Read the model definition and answer for the solid it produces. Units are mm, in the model's axes. A direction names the side the tool comes from. Give positions to 0.01 mm unless a question says otherwise; leave off trailing zeros. Order: outer loops, then holes, each group sorted by start corner. A loop starts at its lowest first (then second) coordinate and runs counter-clockwise, first axis right, second up. Notation, with made-up numbers: (83, 4.25) -> (106, 4.25) arc R27 ccw to (106, 40.25) -> close; hole circle Ø11 at (50.25, 14). An arc over 180 degrees is marked (long way). Use one line per item in the form item = value.
```python
from build123d import *

# Parameters (mm, degrees)
F0_W        = 22
F0_H        = 2
F1_DEPTH    = 25
F2_T1_DEPTH = 25
F2_T3_DEPTH = 35.98872287
F2_T5_DEPTH = 34.5227248018
F2_T7_DEPTH = 35


# Not quite as in the source:
# - a fillet or chamfer that OpenCascade refuses, or shapes differently, is made with other operations: its cross-section is extruded or revolved along the edge and cut away or added


with BuildPart() as f1:
    # F0 (on Top) → F1 (new body)
    with BuildSketch(Plane.XY):
        with BuildLine():
            ThreePointArc((-4.8733971724, -18.3643676722), (-18.9479647202, 1.4052163402), (-2.1111111111, 18.88235181))
            Line((-2.1111111111, 18.88235181), (-2.5, 22.360679775))
            ThreePointArc((-2.5, 22.360679775), (-21.7874934858, 5.6173950908), (-13, -18.3643676722))
            Line((-13, -18.3643676722), (-4.8733971724, -18.3643676722))
        make_face()
        with BuildLine():
            ThreePointArc((2.1111111111, 18.88235181), (14.1617638575, 12.6666666667), (19, 0))
            ThreePointArc((19, 0), (15.0597899434, -11.5845900602), (4.8733971724, -18.3643676722))
            Line((4.8733971724, -18.3643676722), (13, -18.3643676722))
            ThreePointArc((13, -18.3643676722), (19.9843688917, -10.3380365641), (22.5, 0))
            ThreePointArc((22.5, 0), (16.7705098312, 15), (2.5, 22.360679775))
            Line((2.5, 22.360679775), (2.1111111111, 18.88235181))
        make_face()
        with BuildLine():
            Line((13, -18.3643676722), (4.8733971724, -18.3643676722))
            ThreePointArc((4.8733971724, -18.3643676722), (0, -19), (-4.8733971724, -18.3643676722))
            Line((-4.8733971724, -18.3643676722), (-13, -18.3643676722))
            ThreePointArc((-13, -18.3643676722), (0, -22.5), (13, -18.3643676722))
        make_face()
        with BuildLine():
            Line((13, -26.3643676722), (13, -18.3643676722))
            ThreePointArc((13, -18.3643676722), (0, -22.5), (-13, -18.3643676722))
            Line((-13, -18.3643676722), (-13, -26.3643676722))
            Line((-13, -26.3643676722), (13, -26.3643676722))
        make_face()
        with Locations((0, -23.5643676722)):
            Rectangle(F0_W, F0_H, mode=Mode.SUBTRACT)
    extrude(amount=F1_DEPTH)

    # F2: fillet of radius 2 on 8 edges, made by hand

    # F2_s2 → F2_t1 (join)
    with BuildSketch(Plane.XY):
        with BuildLine():
            ThreePointArc((-13.7755102041, -17.79003425), (-13.2043135586, -18.490740056), (-13, -19.3713706278))
            Line((-13, -19.3713706278), (-13, -18.3643676722))
            ThreePointArc((-13, -18.3643676722), (-13.390834604, -18.0813591471), (-13.7755102041, -17.79003425))
        make_face()
        with BuildLine():
            ThreePointArc((13, -19.3713706278), (13.2043135586, -18.490740056), (13.7755102041, -17.79003425))
            ThreePointArc((13.7755102041, -17.79003425), (13.390834604, -18.0813591471), (13, -18.3643676722))
            Line((13, -18.3643676722), (13, -19.3713706278))
        make_face()
    extrude(amount=F2_T1_DEPTH)

    # F2_s4 → F2_t3 (cut)
    with BuildSketch(Plane.XY.offset(-5.494361435)):
        with BuildLine():
            ThreePointArc((-2.2669117515, 20.275875101), (-3.0840105352, 21.6753462818), (-4.6696036077, 22.0101068182))
            ThreePointArc((-4.6696036077, 22.0101068182), (-3.5890847472, 22.2118993037), (-2.5, 22.360679775))
            Line((-2.5, 22.360679775), (-2.2669117515, 20.275875101))
        make_face()
        with BuildLine():
            ThreePointArc((2.2669117515, 20.275875101), (3.0840105352, 21.6753462818), (4.6696036077, 22.0101068182))
            ThreePointArc((4.6696036077, 22.0101068182), (3.5890847472, 22.2118993037), (2.5, 22.360679775))
            Line((2.5, 22.360679775), (2.2669117515, 20.275875101))
        make_face()
    extrude(amount=F2_T3_DEPTH, mode=Mode.SUBTRACT)

    # F2_s6 → F2_t5 (cut)
    with BuildSketch(Plane.XY.offset(-4.7613624009)):
        with BuildLine():
            ThreePointArc((-2.3227272178, 20.7751038089), (-2.6900167457, 19.3804728744), (-3.8998343218, 18.5954642927))
            ThreePointArc((-3.8998343218, 18.5954642927), (-3.0088938767, 18.7602387415), (-2.1111111111, 18.88235181))
            Line((-2.1111111111, 18.88235181), (-2.3227272178, 20.7751038089))
        make_face()
        with BuildLine():
            ThreePointArc((3.8998343218, 18.5954642927), (2.6900167457, 19.3804728744), (2.3227272178, 20.7751038089))
            Line((2.3227272178, 20.7751038089), (2.1111111111, 18.88235181))
            ThreePointArc((2.1111111111, 18.88235181), (3.0088938767, 18.7602387415), (3.8998343218, 18.5954642927))
        make_face()
    extrude(amount=F2_T5_DEPTH, mode=Mode.SUBTRACT)

    # F2_s8 → F2_t7 (cut)
    with BuildSketch(Plane.XY.offset(-5)):
        with BuildLine():
            ThreePointArc((11, -26.3643676722), (12.4142135624, -25.7785812346), (13, -24.3643676722))
            Line((13, -24.3643676722), (13, -26.3643676722))
            Line((13, -26.3643676722), (11, -26.3643676722))
        make_face()
        with BuildLine():
            ThreePointArc((-13, -24.3643676722), (-12.4142135624, -25.7785812346), (-11, -26.3643676722))
            Line((-11, -26.3643676722), (-13, -26.3643676722))
            Line((-13, -26.3643676722), (-13, -24.3643676722))
        make_face()
    extrude(amount=F2_T7_DEPTH, mode=Mode.SUBTRACT)


solid = f1.part
```
Item 1: Given pin 1 Ø10 at (y, z) = (10, 4) entering from +X; pin 2 Ø6 at (x, z) = (-12, 14) entering from +Y; pin 3 Ø1 at (x, z) = (16.5, 3) entering from -Y, each flat-ended and moving along its own axis, determine where each tip first touches the part or whether it passes through.
Checks:
pin_1 = 21.94
pin_2 = 20.62
pin_3 = -15.82
Item 2: Determine the mould class of faces 4 (the flat face through (13, -22, 12)), 5 (the flat face through (-10.1, -16.4, 0)), 6 (the cylindrical face through (-2.755, 19.295, 12.325)) for opening direction X: +X half, -X half, draft (parallel to the pull), parting line (faces both ways), or undercut.
Checks:
face_4 = +X half
face_5 = draft
face_6 = undercut
Item 3: Which of the six approach directions +Z, -Z, +X, -X, +Y, -Y give full straight-line access (tool end or side, diameter ignored) to faces 1 (the flat face through (-13, -22, 12)), 2 (the cylindrical face through (3.17, 21.734, 12.325)), 3 (the flat face through (11, -24, 12))?
Checks:
face_1 = +Z, -Z, -X, -Y
face_2 = +Z, -Z, +Y
face_3 = +Z, -Z
Item 4: The part is cut by section C-C on z = 9.75. Give the vertices of the cut face in (x, y).
Checks:
outline = (-13.78, -17.79) arc R2 cw to (-13, -19.37) -> (-13, -24.36) arc R2 ccw to (-11, -26.36) -> (11, -26.36) arc R2 ccw to (13, -24.36) -> (13, -19.37) arc R2 cw to (13.78, -17.79) arc R22.5 ccw to (4.67, 22.01) arc R2 ccw to (2.31, 20.52) arc R2 ccw to (3.9, 18.6) arc R19 cw (long way) to (-3.9, 18.6) arc R2 ccw to (-2.31, 20.52) arc R2 ccw to (-4.67, 22.01) arc R22.5 ccw to start; hole (-11, -24.56) -> (11, -24.56) -> (11, -22.56) -> (-11, -22.56) -> close
Item 5: The part is cut by section A-A on x = 0. Give the vertices of the cut face in (y, z).
Checks:
outline = (-26.36, 0) -> (-24.56, 0) -> (-24.56, 25) -> (-26.36, 25) -> close; (-22.56, 0) -> (-19, 0) -> (-19, 25) -> (-22.56, 25) -> close
Item 6: Straight lines are drawn through the part: L1, parallel to Y at x = -5, z = 6.75; L2, parallel to Y at x = -4.5, z = 10.75; L3, parallel to Y at x = -0.5, z = 1. For each, find the intervals that lie inside material, in ascending order. Write a range as from..to.
Checks:
L1 = -26.36..-24.56, -22.56..-18.33, 18.33..21.94
L2 = -26.36..-24.56, -22.56..-18.46, 18.46..22.04
L3 = -26.36..-24.56, -22.56..-18.99
Item 7: The part is cut by section B-B on y = 3.5. Give the vertices of the cut face in (x, z).
Checks:
outline = (-22.23, 0) -> (-18.67, 0) -> (-18.67, 25) -> (-22.23, 25) -> close; (18.67, 0) -> (22.23, 0) -> (22.23, 25) -> (18.67, 25) -> close
Item 8: The part is cut by section D-D on x = -20. Give the vertices of the cut face in (y, z), and give its area (3 significant figures).
Checks:
outline = (-10.31, 0) -> (10.31, 0) -> (10.31, 25) -> (-10.31, 25) -> close
area = 515 mm²
